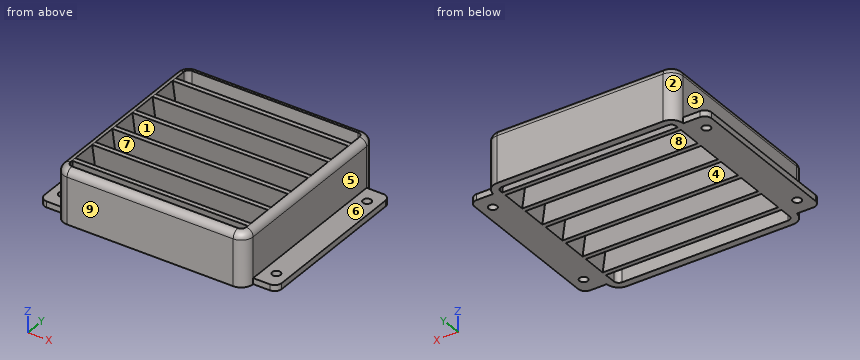
```python
from build123d import *

# Parameters (mm, degrees)
PAD_DEPTH           = 2.5
FILLET_R            = 3
SKETCH002_R         = 1.75
POCKET_DEPTH        = 0.001
POCKET_DEPTH_BACK   = -2.501
PAD001_DEPTH        = 20
FILLET001_R         = 2.9
PAD002_DEPTH        = 74
LINEARPATTERN_COUNT = 6
LINEARPATTERN_PITCH = 12.4


with BuildPart() as part:
    # Sketch001 → Pad (new body)
    with BuildSketch(Plane.XY):
        with BuildLine():
            Line((-50, 35), (-40, 35))
            ThreePointArc((-35, 40), (-38.535534, 38.535534), (-40, 35))
            Line((-35, 40), (35, 40))
            ThreePointArc((40, 35), (38.535534, 38.535534), (35, 40))
            Line((40, 35), (50, 35))
            Line((50, 35), (50, -35))
            Line((50, -35), (40, -35))
            ThreePointArc((35, -40), (38.535534, -38.535534), (40, -35))
            Line((35, -40), (-35, -40))
            ThreePointArc((-40, -35), (-38.535534, -38.535534), (-35, -40))
            Line((-50, -35), (-40, -35))
            Line((-50, 35), (-50, -35))
        make_face()
        with BuildLine():
            ThreePointArc((-35, 37), (-36.414214, 36.414214), (-37, 35))
            Line((-37, -35), (-37, 35))
            ThreePointArc((-37, -35), (-36.414214, -36.414214), (-35, -37))
            Line((35, -37), (-35, -37))
            ThreePointArc((35, -37), (36.414214, -36.414214), (37, -35))
            Line((37, 35), (37, -35))
            ThreePointArc((37, 35), (36.414214, 36.414214), (35, 37))
            Line((-35, 37), (35, 37))
        make_face(mode=Mode.SUBTRACT)
    extrude(amount=PAD_DEPTH)

    # Fillet
    fillet_edges = [part.edges().sort_by_distance(p)[0] for p in [
        (-50, -35, 1.25),
        (50, -35, 1.25),
        (-50, 35, 1.25),
        (50, 35, 1.25),
    ]]
    fillet(fillet_edges, radius=FILLET_R)

    # Sketch002 → Pocket (cut, two sides)
    with BuildSketch(Plane.XY) as pocket_sk:
        with Locations((-45, 28)):
            Circle(SKETCH002_R)
        with Locations((-45, -28)):
            Circle(SKETCH002_R)
        with Locations((45, -28)):
            Circle(SKETCH002_R)
        with Locations((45, 28)):
            Circle(SKETCH002_R)
    extrude(amount=-POCKET_DEPTH, mode=Mode.SUBTRACT)
    extrude(pocket_sk.sketch, amount=-POCKET_DEPTH_BACK, mode=Mode.SUBTRACT)

    # Sketch003 → Pad001 (join)
    with BuildSketch(Plane.XY.offset(2.5)):
        with BuildLine():
            ThreePointArc((-35, 40), (-38.535534, 38.535534), (-40, 35))
            Line((-40, -35), (-40, 35))
            ThreePointArc((-40, -35), (-38.535534, -38.535534), (-35, -40))
            Line((35, -40), (-35, -40))
            ThreePointArc((35, -40), (38.535534, -38.535534), (40, -35))
            Line((40, 35), (40, -35))
            ThreePointArc((40, 35), (38.535534, 38.535534), (35, 40))
            Line((-35, 40), (35, 40))
        make_face()
        with BuildLine():
            ThreePointArc((-35, 37), (-36.414214, 36.414214), (-37, 35))
            Line((-37, -35), (-37, 35))
            ThreePointArc((-37, -35), (-36.414214, -36.414214), (-35, -37))
            Line((35, -37), (-35, -37))
            ThreePointArc((35, -37), (36.414214, -36.414214), (37, -35))
            Line((37, 35), (37, -35))
            ThreePointArc((37, 35), (36.414214, 36.414214), (35, 37))
            Line((-35, 37), (35, 37))
        make_face(mode=Mode.SUBTRACT)
    extrude(amount=PAD001_DEPTH)

    # Fillet001
    fillet001_edges = [part.edges().sort_by_distance(p)[0] for p in [
        (0, 40, 22.5),
    ]]
    fillet(fillet001_edges, radius=FILLET001_R)

    # Sketch004 → Pad002 (join)
    with BuildSketch(Plane.YZ.offset(-37)):
        Polygon((33.967357, 0), (30, 22.5), (28, 22.5), (31.967357, 0), align=None)
    pad002 = extrude(amount=PAD002_DEPTH)

    # LinearPattern: Pad002 ×6
    with Locations(*[(0, -i * LINEARPATTERN_PITCH, 0) for i in range(1, LINEARPATTERN_COUNT)]):
        add(pad002)


solid = part.part
```
Geometry check sheet. Reference: the model listing, model coordinates, mm. Face numbers are marked on the shaded views. A direction names the side the tool comes from. Coordinates: 2 decimals unless noted, no trailing zeros. Order: outer loops, then holes, each group sorted by start corner. A loop starts at its lowest first (then second) coordinate and runs counter-clockwise, first axis right, second up. Notation, with made-up numbers: M -4,71 L 11,71 A18 ccw 11,91 Z; hole C -18.75,6 d8. An arc over 180 degrees is marked long. Answer as a JSON object with one key per item and string values.
Q1. Scan lines: line 1 (Y direction, x = -45, z = 0.95); line 2 (X direction, y = 28, z = 1.55); line 3 (X direction, y = 11.5, z = 6). Record each from-to range of solid material in increasing order.
Results are:
{"line 1": "y = -35 to -29.75, -26.25 to 26.25, 29.75 to 35", "line 2": "x = -50 to -46.75, -43.25 to -37, 37 to 43.25, 46.75 to 50", "line 3": "x = -40 to -37, 37 to 40"}
Q2. Cross-section at A-A on x = 31.5. Give the number of separate pieces and of enclosed holes in the cut face, and give its area (3 significant figures).
Results are:
{"separate pieces": "8", "enclosed holes": "0", "area": "401 mm²"}
Q3. Release check for a two-part mould opening along Y. For the marked faces 6, 7, 8 and 9 record: released by +Y, released by -Y, zero draft, split by the parting line, or undercut.
Results are:
{"face 6": "zero draft", "face 7": "undercut", "face 8": "undercut", "face 9": "released by -Y"}
Q4. Tool access check on the marked faces 1, 2, 3, 4 and 5. Record the directions out of +Z, -Z, +X, -X, +Y, -Y that give a thin tool (end or side, any length) a straight path to the whole face; none if there is none.
Results are:
{"face 1": "-Z", "face 2": "+Z, -Z, -X, +Y", "face 3": "+Z, -X, +Y, -Y", "face 4": "+Z", "face 5": "+Z, +X, +Y, -Y"}
Q5. Cross-section at B-B on x = 45. Record the cut outline in (y, z).
Results are:
{"outline": "M -35,0 L -29.75,0 L -29.75,2.5 L -35,2.5 Z; M -26.25,0 L 26.25,0 L 26.25,2.5 L -26.25,2.5 Z; M 29.75,0 L 35,0 L 35,2.5 L 29.75,2.5 Z"}
Q6. Depth check by flat-ended pin: pin 1 Ø0.8 at (x, z) = (44, 0.5) entering from -Y; pin 2 Ø3 at (y, z) = (-32, 20) entering from -X; pin 3 Ø1.5 at (y, z) = (-32.5, 6) entering from +X. Enter the tip coordinate at first touch or a pass-through.
Results are:
{"pin 1": "stops at y = -35", "pin 2": "stops at x = -40", "pin 3": "stops at x = 40"}
